Source: three-view drawing plus pictorial views. Frame: mm from the lowest corner of the part. Round coordinates to 2 decimals unless told otherwise and drop trailing zeros. Write each loop counter-clockwise with the first axis right and the second up, starting at its lowest first coordinate (ties: lowest second). Pieces come first, ordered by that corner, then holes. Notation, with made-up numbers: M 36.5,10 L 89.5,10 A21 ccw 89.5,22 Z; hole C -9,-13 d11. An arc over 180 degrees is marked long. Put each result on its own line as item: value. Start each with the question number.
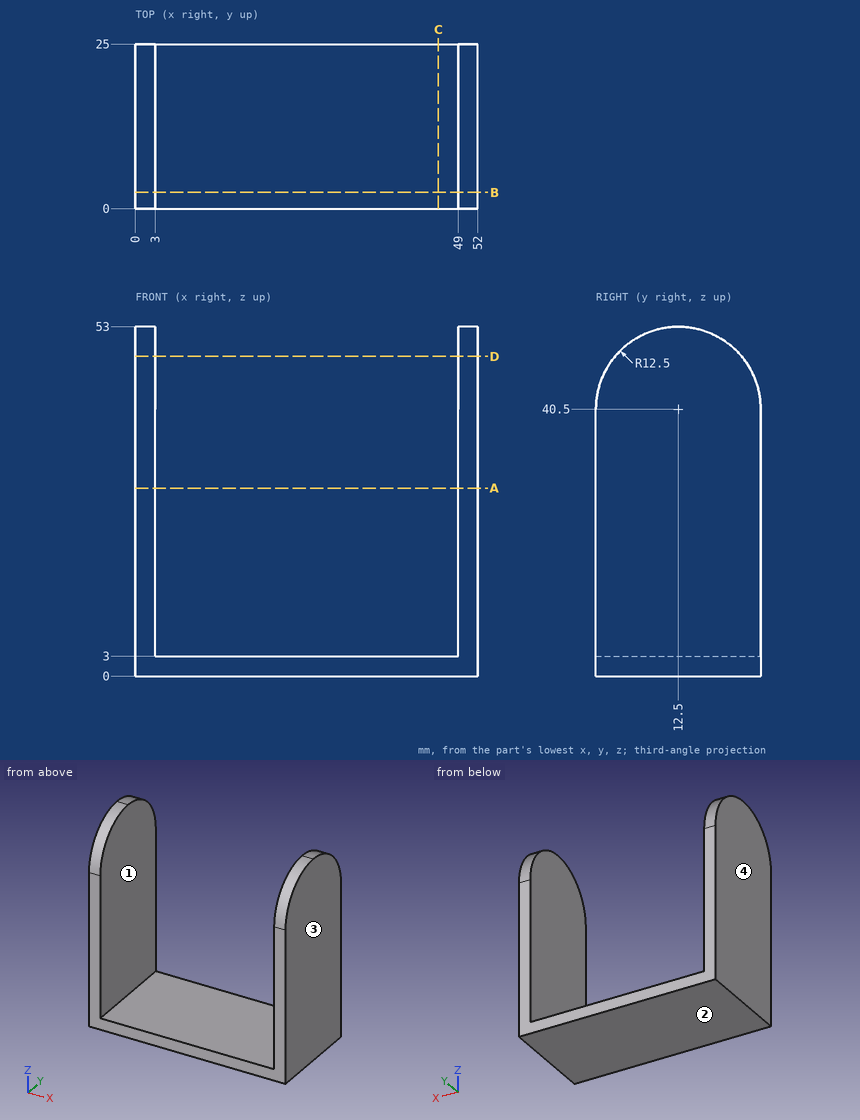
(1) Ray query, line 1 along X through (y, z) = (17.25, 37.5); line 2 along Z through (x, y) = (29, 20.75). Return the intervals inside material, ascending.
(2) Section query D-D (z = 48.5). Return loops of the section in (x, y).
(3) Section query A-A (z = 28.5). Return loops of the section in (x, y), and give its area (3 significant figures).
(4) Contact query for a flat-ended pin moving along its axis: P1, Ø8, axis at x = 17, y = 14.5, coming from the +Z side. Output: stop coordinate, or through.
(5) Pull-direction query (X, two-part tool) for the marked faces 1, 2, 3 and 4; classes: +X half, -X half, draft (parallel to the pull), parting line (faces both ways), or undercut.
(6) Section query B-B (y = 2.5). Return loops of the section in (x, z).
(7) Section query C-C (x = 46). Return loops of the section in (y, z).
Entries:
1. line 1: 0 to 3, 49 to 52
1. line 2: 0 to 3
2. outline: M 0,2.9 L 3,2.9 L 3,22.1 L 0,22.1 Z; M 49,2.9 L 52,2.9 L 52,22.1 L 49,22.1 Z
3. outline: M 0,0 L 3,0 L 3,25 L 0,25 Z; M 49,0 L 52,0 L 52,25 L 49,25 Z
3. area: 150 mm2
4. P1: z = 3
5. face 1: undercut
5. face 2: draft
5. face 3: +X half
5. face 4: -X half
6. outline: M 0,0 L 52,0 L 52,48 L 49,48 L 49,3 L 3,3 L 3,48 L 0,48 Z
7. outline: M 0,0 L 25,0 L 25,3 L 0,3 Z
